```python
from build123d import *

# Parameters (mm, degrees)
F0_R      = 12.6
F0_R_2    = 6.75
F1_DEPTH  = 30
F2_W      = 11
F2_H      = 13
F3_DEPTH  = 15
F5_W      = 1.3
F5_H      = 5
F6_DEPTH  = 12.5
F7_W      = 1.5
F7_H      = 5
F8_DEPTH  = 12.5
F10_DEPTH = 10
F12_DEPTH = 5


with BuildPart() as f1:
    # F0 (on Top) → F1 (new body)
    with BuildSketch(Plane.XY):
        Circle(F0_R)
        Circle(F0_R_2, mode=Mode.SUBTRACT)
    extrude(amount=F1_DEPTH)


with BuildPart() as f3:
    # F2 (on Right) → F3 (new body, symmetric)
    with BuildSketch(Plane.YZ):
        with Locations((0, 6.5)):
            Rectangle(F2_W, F2_H)
    extrude(amount=F3_DEPTH, both=True)


with BuildPart() as f1_1:
    add(f1.part)

    # F4: cut F3
    add(f3.part, mode=Mode.SUBTRACT)

    # F5 (on Right) → F6 (cut, symmetric)
    with BuildSketch(Plane.YZ):
        with Locations((-11.95, 6.7)):
            Rectangle(F5_W, F5_H)
    extrude(amount=F6_DEPTH, both=True, mode=Mode.SUBTRACT)

    # F7 (on Right) → F8 (cut, symmetric)
    with BuildSketch(Plane.YZ):
        with Locations((11.85, 6.7)):
            Rectangle(F7_W, F7_H)
    extrude(amount=F8_DEPTH, both=True, mode=Mode.SUBTRACT)

    # F9 (on face) → F10 (join)
    with BuildSketch(Plane.XY.offset(30)):
        with BuildLine():
            Line((-12.0290273921, 3.75), (-22.5, 3.75))
            Line((-22.5, 3.75), (-22.5, -3.75))
            Line((-22.5, -3.75), (-12.0290273921, -3.75))
            ThreePointArc((-12.0290273921, -3.75), (-12.6, 0), (-12.0290273921, 3.75))
        make_face()
        with BuildLine():
            Line((22.5, 3.75), (12.0290273921, 3.75))
            ThreePointArc((12.0290273921, 3.75), (12.4564390004, 1.8966094563), (12.6, 0))
            ThreePointArc((12.6, 0), (12.4564390004, -1.8966094563), (12.0290273921, -3.75))
            Line((12.0290273921, -3.75), (22.5, -3.75))
            Line((22.5, -3.75), (22.5, 3.75))
        make_face()
    extrude(amount=-F10_DEPTH)

    # F11 (on face) → F12 (join)
    with BuildSketch(Plane.XY.offset(30)):
        with BuildLine():
            ThreePointArc((-18.984, -3.75), (-16.3323495706, -2.6516504294), (-15.234, 0))
            ThreePointArc((-15.234, 0), (-16.3323495706, 2.6516504294), (-18.984, 3.75))
            ThreePointArc((-18.984, 3.75), (-21.1255820463, 3.0783317461), (-22.5, 1.3039340474))
            Line((-22.5, 1.3039340474), (-22.5, -1.3039340474))
            ThreePointArc((-22.5, -1.3039340474), (-21.1255820463, -3.0783317461), (-18.984, -3.75))
        make_face()
        with BuildLine():
            ThreePointArc((22.5, 1.3048106807), (21.1255234866, 3.0785987115), (18.9843252301, 3.75))
            ThreePointArc((18.9843252301, 3.75), (15.2343252301, 0), (18.9843252301, -3.75))
            ThreePointArc((18.9843252301, -3.75), (21.1255234866, -3.0785987115), (22.5, -1.3048106807))
            Line((22.5, -1.3048106807), (22.5, 1.3048106807))
        make_face()
    extrude(amount=F12_DEPTH)


solid = f1_1.part
```
For this review, take the finished solid that the model builds, in its own axes (mm). A direction names the side the tool comes from. Coordinates: 2 decimals unless noted, no trailing zeros. Write each loop counter-clockwise with the first axis right and the second up, starting at its lowest first coordinate (ties: lowest second). Pieces come first, ordered by that corner, then holes.
(1) For pin 1 Ø1.4 at (x, y) = (1.5, -12) entering from +Z; pin 2 Ø4 at (x, z) = (9, 29) entering from +Y; pin 3 Ø8.5 at (x, y) = (19, 0.5) entering from -Z; pin 4 Ø1 at (y, z) = (2.5, 11.5) entering from -X, all flat-tipped, find the tip position at first contact; note any pin that passes through.
(2) Add section B-B on z = 24.5. Give the boundary of the cut face in (x, y).
(3) The part is to be moulded in two halves that separate along Y. For faces 4 (the face through (-8, -5.5, 6)), 5 (the face through (17, 3.75, 25)), 6 (the face through (-22, -3, 30)), say which applies: +Y half, -Y half, draft (parallel to the pull), parting line (faces both ways), or undercut.
(4) Add section A-A on x = 0. Give the boundary of the cut face in (y, z).
(5) Add section D-D on x = -9. Give the boundary of the cut face in (y, z), then the cut area to 3 significant figures.
(6) Wall thickness on probe 1 along Y at (x, z) = (0, 22); probe 2 along Y at (x, z) = (0, 6.25); probe 3 along Z at (x, y) = (-0.5, 8.5): over which ranges is each line inside the solid? List them lowest first.
(7) Tool access review of faces 1 (the face through (0, 12, 4.2)), 2 (the face through (0, -12, 9.2)), 3 (the face through (-8, 5.5, 6)): name each direction out of +Z, -Z, +X, -X, +Y, -Y from which nothing blocks a thin tool from reaching the whole face with its end or side.
(8) Add section C-C on z = 33.5. Give the boundary of the cut face in (x, y).
Answer sheet:
1. pin 1: stops at z = 30
1. pin 2: stops at y = 10.48
1. pin 3: stops at z = 20
1. pin 4: passes through
2. outline: (-22.5, -3.75) - (-12.03, -3.75) arc R12.6 ccw to (12.03, -3.75) - (22.5, -3.75) - (22.5, 3.75) - (12.03, 3.75) arc R12.6 ccw to (-12.03, 3.75) - (-22.5, 3.75) - close; hole circle Ø13.5 at (0, 0)
3. face 4: undercut
3. face 5: +Y half
3. face 6: draft
4. outline: (-12.6, 0) - (-6.75, 0) - (-6.75, 30) - (-12.6, 30) - (-12.6, 9.2) - (-11.3, 9.2) - (-11.3, 4.2) - (-12.6, 4.2) - close; (6.75, 0) - (12.6, 0) - (12.6, 4.2) - (11.1, 4.2) - (11.1, 9.2) - (12.6, 9.2) - (12.6, 30) - (6.75, 30) - close
5. outline: (-8.82, 0) - (-5.5, 0) - (-5.5, 13) - (5.5, 13) - (5.5, 0) - (8.82, 0) - (8.82, 30) - (-8.82, 30) - close
5. area: 386 mm2
6. probe 1: y = -12.6 to -6.75, 6.75 to 12.6
6. probe 2: y = -11.3 to -6.75, 6.75 to 11.1
6. probe 3: z = 0 to 30
7. face 1: +X, -X, +Y
7. face 2: +X, -X, -Y
7. face 3: -Z, +X, -X
8. outline: (-22.5, -1.3) arc R3.75 ccw (long way) to (-22.5, 1.3) - close; (22.5, -1.3) - (22.5, 1.3) arc R3.75 ccw (long way) to start
